```python
from build123d import *

# Parameters (mm, degrees)
BOSS_EXTRUDE1_DEPTH = 20
SKETCH4_R           = 2.6
CUT_EXTRUDE1_DEPTH  = 42.231056256
CUT_EXTRUDE2_DEPTH  = 3
CUT_EXTRUDE3_DEPTH  = 8
SKETCH7_R           = 2.6
CUT_EXTRUDE4_DEPTH  = 42.231056256
FILLET1_R           = 5


with BuildPart() as part:
    # Sketch1 → Boss-Extrude1 (new body)
    with BuildSketch(Plane(origin=(0, 0, 0), x_dir=(1, 0, 0), z_dir=(0, 1, 0))):
        Polygon((0, 0), (0, 30), (-20, 30), (-20, -30), (0, -30), align=None)
    extrude(amount=BOSS_EXTRUDE1_DEPTH)

    # Sketch4 → Cut-Extrude1 (cut, through all)
    with BuildSketch(Plane(origin=(0, 20, 0), x_dir=(1, 0, 0), z_dir=(0, 1, 0))):
        with Locations(Location((-10, 0, 0), (0, 0, 270))):
            Circle(SKETCH4_R)
    extrude(amount=-CUT_EXTRUDE1_DEPTH, mode=Mode.SUBTRACT)

    # Sketch5 → Cut-Extrude2 (cut)
    with BuildSketch(Plane(origin=(0, 20, 0), x_dir=(1, 0, 0), z_dir=(0, 1, 0))):
        Polygon((-10, 4.67653718), (-14.05, 2.33826859), (-14.05, -2.33826859), (-10, -4.67653718), (-5.95, -2.33826859), (-5.95, 2.33826859), align=None)
    extrude(amount=-CUT_EXTRUDE2_DEPTH, mode=Mode.SUBTRACT)

    # Sketch6 → Cut-Extrude3 (cut)
    with BuildSketch(Plane.XZ):
        Polygon((-10, -4.67653718), (-5.95, -2.33826859), (-5.95, 2.33826859), (-10, 4.67653718), (-14.05, 2.33826859), (-14.05, -2.33826859), align=None)
    extrude(amount=-CUT_EXTRUDE3_DEPTH, mode=Mode.SUBTRACT)

    # Sketch7 → Cut-Extrude4 (cut, through all)
    with BuildSketch(Plane(origin=(0, 0, 0), x_dir=(0, 0, -1), z_dir=(1, 0, 0))):
        with Locations((-20, 10)):
            Circle(SKETCH7_R)
        with Locations((20, 10)):
            Circle(SKETCH7_R)
    extrude(amount=-CUT_EXTRUDE4_DEPTH, mode=Mode.SUBTRACT)

    # Fillet1
    fillet1_edges = [part.edges().sort_by_distance(p)[0] for p in [
        (-20, 10, 30),
        (-20, 10, -30),
    ]]
    fillet(fillet1_edges, radius=FILLET1_R)


solid = part.part
```
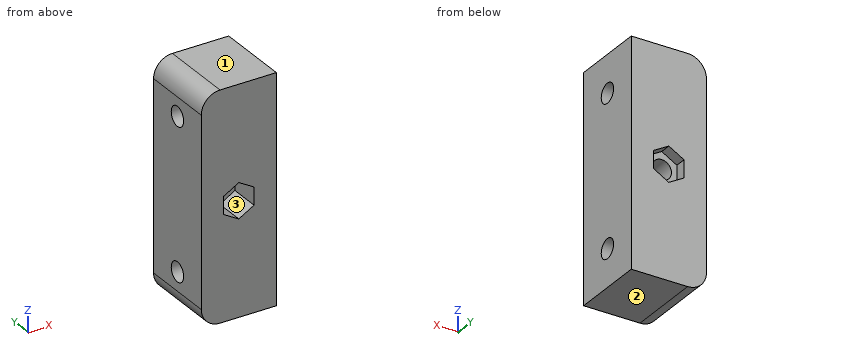
CAD build for the part. Positions are in the model's coordinates, mm. Face numbers are marked on the shaded views. Round coordinates to 2 decimals unless told otherwise and drop trailing zeros. Write each loop counter-clockwise with the first axis right and the second up, starting at its lowest first coordinate (ties: lowest second). Pieces come first, ordered by that corner, then holes. Notation, with made-up numbers: (48.5, 68.25) - (61.5, 68.25) arc R23 cw to (61.5, 95.25) - close; hole circle Ø8 at (-9, -8.5). An arc over 180 degrees is marked (long way). Return JSON: item names as keys, results as strings. Group by question number.
Item 1: Band-saw the part on B-B on x = -11. List the corners of the cut face in (y, z).
Item 2: Band-saw the part on D-D on z = 0. List the corners of the cut face in (x, y).
Item 3: Band-saw the part on C-C on y = 14. List the corners of the cut face in (x, z), plus the area to 3 significant figures.
Item 4: Probe probe 1 along Y at (x, z) = (-7.75, -20); probe 2 along X at (y, z) = (15.25, 0); probe 3 along Z at (x, y) = (-3.75, 8). List the from-to ranges inside material, lowest first.
Item 5: Flat gauge pins, fed straight in: pin 1 Ø4 at (x, z) = (-11, 0) entering from -Y; pin 2 Ø4 at (x, z) = (-11.5, 0) entering from +Y; pin 3 Ø2 at (x, z) = (-14.5, -21) entering from -Y. Where does each tip first touch, or does it go through?
Item 6: Band-saw the part on A-A on y = 10. List the corners of the cut face in (x, z), plus the area to 3 significant figures.
Item 7: Mould opens along Z. For the marked faces 1, 2 and 3 say: +Z half, -Z half, draft (parallel to the pull), parting line (faces both ways), or undercut.
Resolved:
{
 "1": {"outline": "(0, -30) - (20, -30) - (20, -4.1) - (17, -4.1) - (17, -2.4) - (8, -2.4) - (8, -4.1) - (0, -4.1) - close; (0, 4.1) - (8, 4.1) - (8, 2.4) - (17, 2.4) - (17, 4.1) - (20, 4.1) - (20, 30) - (0, 30) - close; hole circle Ø5.2 at (10, -20); hole circle Ø5.2 at (10, 20)"},
 "2": {"outline": "(-20, 0) - (-14.05, 0) - (-14.05, 8) - (-12.6, 8) - (-12.6, 17) - (-14.05, 17) - (-14.05, 20) - (-20, 20) - close; (-7.4, 8) - (-5.95, 8) - (-5.95, 0) - (0, 0) - (0, 20) - (-5.95, 20) - (-5.95, 17) - (-7.4, 17) - close"},
 "3": {"outline": "(-20, -25) arc R5 ccw to (-15, -30) - (0, -30) - (0, 30) - (-15, 30) arc R5 ccw to (-20, 25) - close; hole circle Ø5.2 at (-10, 0)", "area": "1,170 mm²"},
 "4": {"probe 1": "y = 0 to 7.4, 12.6 to 20", "probe 2": "x = -20 to -12.6, -7.4 to 0", "probe 3": "z = -30 to -21.66, -18.34 to 18.34, 21.66 to 30"},
 "5": {"pin 1": "stops at y = 8", "pin 2": "stops at y = 17", "pin 3": "stops at y = 0"},
 "6": {"outline": "(-20, -25) arc R5 ccw to (-15, -30) - (0, -30) - (0, -22.6) - (-20, -22.6) - close; (-20, -17.4) - (0, -17.4) - (0, 17.4) - (-20, 17.4) - close; (-20, 22.6) - (0, 22.6) - (0, 30) - (-15, 30) arc R5 ccw to (-20, 25) - close; hole circle Ø5.2 at (-10, 0)", "area": "960 mm²"},
 "7": {"face 1": "+Z half", "face 2": "-Z half", "face 3": "undercut"}
}
